Here's how the part is built. I have some questions about the finished solid (model axes, mm). A direction names the side the tool comes from. Round coordinates to 2 decimals unless told otherwise and drop trailing zeros. Order: outer loops, then holes, each group sorted by start corner. A loop starts at its lowest first (then second) coordinate and runs counter-clockwise, first axis right, second up. Notation, with made-up numbers: (60.5, 25.25) -> (112.5, 25.25) arc R11 ccw to (112.5, 46.25) -> close; hole circle Ø5 at (32, 73.25). An arc over 180 degrees is marked (long way). Use a Markdown table: item, result. Add a question column.
(1) On a 3-axis mill with a long thin cutter (end or side, diameter ignored), from which of +Z, -Z, +X, -X, +Y, -Y can I reach the whole of each face in a straight line? I mean faces 1 (the face through (-2, -3, -2.35)), 2 (the face through (2, -3, -2.35)), 3 (the face through (0, -3.962, -3)). Say none if no direction works.
(2) I'm going to push flat-ended pins straight in: P1, Ø1.4, axis at x = 1.5, y = -3, coming from the -Z side; P2, Ø1.5, axis at y = 1.5, z = 4, coming from the -X side. Where does each tip first touch, or does it pass through?
(3) Thinking about a two-plate mould opening in Y: for faces 4 (the face through (0, -4.343, 0)), 5 (the face through (-2, 3, -2.35)), 6 (the face through (0.5, -0.1, -1.968)), which applies, pulls with the +Y half, pulls with the -Y half, needs draft (parallel to the pull), parting line crosses it, or undercut?
(4) I want a section at A-A, the plane y = -1. Please give me the cut outline in (x, z), then the cut area to 3 significant figures.
(5) I want a section at D-D, the plane y = 2. Please give me the cut outline in (x, z).
(6) I want a section at B-B, the plane x = 1.75. Please give me the cut outline in (y, z).
(7) I want a section at C-C, the plane z = 6. Please give me the cut outline in (x, y), then the cut area to 3 significant figures.
(8) If I drill on probe 1 along Y at (x, z) = (-0.1, -3.75); probe 2 along Y at (x, z) = (-0.35, -3); probe 3 along X at (y, z) = (1.75, 3), over which ranges is the centre line in solid material (lowest first)?
from build123d import *

# Parameters (mm, degrees)
F0_W           = 4.572
F0_H           = 8.6868
F1_DEPTH       = 2.3495
F2_W           = 2.6416
F2_H           = 5.5372
F3_DEPTH       = 0.508
F4_W           = 1.8288
F4_H           = 1.8288
F5_DEPTH       = 9.525
F7_DEPTH       = 12.7
F9_DEPTH       = 0.381
F11_DEPTH      = 4.3434
F11_DEPTH_BACK = 4.3434
F12_W          = 2.2606
F12_H          = 7.9248
F13_DEPTH      = 2.8966
F14_W          = 0.3048
F14_H          = 0.508
F15_DEPTH      = 3.429


with BuildPart() as f1:
    # F0 (on Top) → F1 (new body, symmetric)
    with BuildSketch(Plane.XY):
        Rectangle(F0_W, F0_H)
    extrude(amount=F1_DEPTH, both=True)

    # F2 (on face) → F3 (cut)
    with BuildSketch(Plane.XY.offset(2.3495)):
        Rectangle(F2_W, F2_H)
    extrude(amount=-F3_DEPTH, mode=Mode.SUBTRACT)

    # F4 (on face) → F5 (join)
    with BuildSketch(Plane(origin=(0, 0, -2.3495), x_dir=(1, 0, 0), z_dir=(0, 0, -1))):
        with Locations((0, -1.4224)):
            Rectangle(F4_W, F4_H)
    extrude(amount=-F5_DEPTH)

    # F6 (on Right) → F7 (cut, symmetric)
    with BuildSketch(Plane.YZ):
        Polygon((1.8122021099, 7.1755), (1.0325978901, 7.1755), (1.4224, 6.6675), align=None)
    extrude(amount=F7_DEPTH, both=True, mode=Mode.SUBTRACT)

    # F8 (on face) → F9 (cut)
    with BuildSketch(Plane(origin=(0, 0, -2.3495), x_dir=(1, 0, 0), z_dir=(0, 0, -1))):
        Polygon((1.1303, 3.9624), (-1.1303, 3.9624), (-1.1303, 2.4384), (-2.286, 2.4384), (-2.286, 0), (-2.286, -2.4384), (-1.1303, -2.4384), (-1.1303, -3.9624), (1.1303, -3.9624), (1.1303, -2.4384), (2.286, -2.4384), (2.286, 0), (2.286, 2.4384), (1.1303, 2.4384), align=None)
    extrude(amount=-F9_DEPTH, mode=Mode.SUBTRACT)

    # F10 (on Front) → F11 (join, two sides)
    with BuildSketch(Plane.XZ) as f11_sk:
        with BuildLine():
            Line((0.5334, -3.9677388407), (0.5334, -2.3495))
            Line((0.5334, -2.3495), (-0.5334, -2.3495))
            Line((-0.5334, -2.3495), (-0.5334, -3.9677388407))
            ThreePointArc((-0.5334, -3.9677388407), (-0.5218235078, -4.1000587521), (-0.487445777, -4.2283581899))
            Line((-0.487445777, -4.2283581899), (-0.3168838925, -4.6969731164))
            ThreePointArc((-0.3168838925, -4.6969731164), (-0.2238903816, -4.8181646192), (-0.0782019668, -4.8641))
            Line((-0.0782019668, -4.8641), (0.0782019668, -4.8641))
            ThreePointArc((0.0782019668, -4.8641), (0.2238903816, -4.8181646192), (0.3168838925, -4.6969731164))
            Line((0.3168838925, -4.6969731164), (0.487445777, -4.2283581899))
            ThreePointArc((0.487445777, -4.2283581899), (0.5218235078, -4.1000587521), (0.5334, -3.9677388407))
        make_face()
    extrude(amount=-F11_DEPTH)
    extrude(f11_sk.sketch, amount=F11_DEPTH_BACK)

    # F12 (on face) → F13 (cut, through all)
    with BuildSketch(Plane(origin=(0, 0, -1.9685), x_dir=(1, 0, 0), z_dir=(0, 0, -1))):
        Rectangle(F12_W, F12_H)
    extrude(amount=F13_DEPTH, mode=Mode.SUBTRACT)

    # F14 (on face) → F15 (join)
    with BuildSketch(Plane(origin=(0, 0, -1.9685), x_dir=(1, 0, 0), z_dir=(0, 0, -1))):
        with Locations((0, 1.905)):
            Rectangle(F14_W, F14_H)
        Rectangle(F14_W, F14_H)
        with Locations((0, -1.905)):
            Rectangle(F14_W, F14_H)
    extrude(amount=F15_DEPTH)


solid = f1.part
Taken from the geometry:
| question | item | result |
|---|---|---|
| 1 | face 1 | -Z, -X, +Y, -Y |
| 1 | face 2 | -Z, +X, +Y, -Y |
| 1 | face 3 | -Z |
| 2 | P1 | stops at z = -2.35 |
| 2 | P2 | stops at x = -0.91 |
| 3 | face 4 | pulls with the -Y half |
| 3 | face 5 | needs draft |
| 3 | face 6 | undercut |
| 4 | outline | (-2.29, -1.97) -> (2.29, -1.97) -> (2.29, 2.35) -> (1.32, 2.35) -> (1.32, 1.84) -> (-1.32, 1.84) -> (-1.32, 2.35) -> (-2.29, 2.35) -> close |
| 4 | area | 18.4 mm2 |
| 5 | outline | (-2.29, -1.97) -> (-0.15, -1.97) -> (-0.15, -5.4) -> (0.15, -5.4) -> (0.15, -1.97) -> (2.29, -1.97) -> (2.29, 2.35) -> (1.32, 2.35) -> (1.32, 1.84) -> (0.91, 1.84) -> (0.91, 7.18) -> (-0.91, 7.18) -> (-0.91, 1.84) -> (-1.32, 1.84) -> (-1.32, 2.35) -> (-2.29, 2.35) -> close |
| 6 | outline | (-4.34, -2.35) -> (-2.44, -2.35) -> (-2.44, -1.97) -> (2.44, -1.97) -> (2.44, -2.35) -> (4.34, -2.35) -> (4.34, 2.35) -> (-4.34, 2.35) -> close |
| 7 | outline | (-0.91, 0.51) -> (0.91, 0.51) -> (0.91, 2.34) -> (-0.91, 2.34) -> close |
| 7 | area | 3.34 mm2 |
| 8 | probe 1 | y = -4.34 to -3.96, -2.16 to -1.65, -0.25 to 0.25, 1.65 to 2.16, 3.96 to 4.34 |
| 8 | probe 2 | y = -4.34 to -3.96, 3.96 to 4.34 |
| 8 | probe 3 | x = -0.91 to 0.91 |
